```python
from build123d import *

# Parameters (mm, degrees)
SKETCH1_W           = 30
SKETCH1_H           = 30
BOSS_EXTRUDE1_DEPTH = 5
SKETCH2_W           = 30
SKETCH2_H           = 5
BOSS_EXTRUDE2_DEPTH = 2.5


with BuildPart() as part:
    # Sketch1 → Boss-Extrude1 (new body)
    with BuildSketch(Plane(origin=(0, 0, 0), x_dir=(0, 0, -1), z_dir=(1, 0, 0))):
        Rectangle(SKETCH1_W, SKETCH1_H)
    extrude(amount=BOSS_EXTRUDE1_DEPTH)

    # Sketch2 → Boss-Extrude2 (add, symmetric)
    with BuildSketch(Plane(origin=(0, 0, 0), x_dir=(1, 0, 0), z_dir=(0, 1, 0))):
        with Locations((20, 11.007087783)):
            Rectangle(SKETCH2_W, SKETCH2_H)
        with Locations((20, -11.007087783)):
            Rectangle(SKETCH2_W, SKETCH2_H)
    extrude(amount=BOSS_EXTRUDE2_DEPTH, both=True)


solid = part.part
```
CAD build for the part. Positions are in the model's coordinates, mm. A direction names the side the tool comes from. Round coordinates to 2 decimals unless told otherwise and drop trailing zeros. Order: outer loops, then holes, each group sorted by start corner. A loop starts at its lowest first (then second) coordinate and runs counter-clockwise, first axis right, second up.
Q1. Two-plate mould, pull along Z, no slides. Class faces 4 (the flat face through (35, 0, 11)), 5 (the flat face through (20, 0, 8.507)), 6 (the flat face through (20, 0, -13.507)): pulls with the +Z half, pulls with the -Z half, needs draft (parallel to the pull), parting line crosses it, or undercut.
Q2. Drop flat-ended pins along their axis: pin 1 (6 mm diameter, centred on y = -4.5, z = 7.5, fed in from +X); pin 2 (4 mm diameter, centred on x = 25, z = -11, fed in from -Y); pin 3 (4 mm diameter, centred on x = 18.5, z = 12, fed in from +Y); pin 4 (4 mm diameter, centred on x = 17, y = 0, fed in from -Z). Give the stop position or say it passes through.
Q3. Slice it at A-A (x = 10.5). Write the cut outline in (y, z).
Q4. Which spindle directions (+Z, -Z, +X, -X, +Y, -Y) get a long thin tool onto all of the face, cutting with end or side? Do faces 1 (the flat face through (20, -2.5, -11)), 2 (the flat face through (20, 0, 13.507)), 3 (the flat face through (20, 2.5, 11)). Say none if no direction does.
Q5. Slice it at C-C (y = 2). Write the cut outline in (x, z).
Q6. Slice it at D-D (y = -9). Write the cut outline in (x, z), and give its area (3 significant figures).
Q7. Slice it at B-B (z = -10.25). Write the cut outline in (x, y).
Q8. Wall check: L1, parallel to X at y = 5.5, z = 10.5; L2, parallel to Z at x = 15, y = 1; L3, parallel to Y at x = 18.5, z = -10. Give the ranges that are in metal, low to high.
Results below:
1. face 4: needs draft
1. face 5: undercut
1. face 6: pulls with the -Z half
2. pin 1: stops at x = 35
2. pin 2: stops at y = -2.5
2. pin 3: stops at y = 2.5
2. pin 4: stops at z = -13.51
3. outline: (-2.5, -13.51) - (2.5, -13.51) - (2.5, -8.51) - (-2.5, -8.51) - close; (-2.5, 8.51) - (2.5, 8.51) - (2.5, 13.51) - (-2.5, 13.51) - close
4. face 1: +Z, -Z, +X, -Y
4. face 2: +Z, +X, +Y, -Y
4. face 3: +Z, -Z, +X, +Y
5. outline: (0, -15) - (5, -15) - (5, -13.51) - (35, -13.51) - (35, -8.51) - (5, -8.51) - (5, 8.51) - (35, 8.51) - (35, 13.51) - (5, 13.51) - (5, 15) - (0, 15) - close
6. outline: (0, -15) - (5, -15) - (5, 15) - (0, 15) - close
6. area: 150 mm2
7. outline: (0, -15) - (5, -15) - (5, -2.5) - (35, -2.5) - (35, 2.5) - (5, 2.5) - (5, 15) - (0, 15) - close
8. L1: x = 0 to 5
8. L2: z = -13.51 to -8.51, 8.51 to 13.51
8. L3: y = -2.5 to 2.5
